Work out the finished part from the listing and answer in its coordinate system (mm). Face numbers are marked on the shaded views. Round coordinates to 2 decimals unless told otherwise and drop trailing zeros. Loops run counter-clockwise (first coordinate to the right, second up) from the corner with the lowest first, then second, coordinate; pieces in that order, holes last. Notation, with made-up numbers: (69.5, -38.5) -> (107.5, -38.5) arc R19 ccw to (107.5, -33.5) -> close; hole circle Ø11 at (9.25, 20.25). An arc over 180 degrees is marked (long way). Use one line per item in the form item = value.
```python
from build123d import *

# Parameters (mm, degrees)
BASE_FLANGE1_DEPTH = 1.524


# Sheet-metal steps are written as plain solids
with BuildPart() as part:
    # Sketch1 → Base-Flange1 (new body)
    with BuildSketch(Plane.XY):
        with BuildLine():
            Line((231.694733782, 24.263932463), (226.322343195, 34.826415896))
            Line((226.322343195, 34.826415896), (224.963957286, 34.135500761))
            Line((224.963957286, 34.135500761), (230.310366707, 23.62409806))
            ThreePointArc((230.310366707, 23.62409806), (229.903279587, 23.531939933), (229.489552508, 23.476777012))
            ThreePointArc((229.489552508, 23.476777012), (228.197526273, 23.373669283), (226.906388141, 23.487358857))
            ThreePointArc((226.906388141, 23.487358857), (226.4596517, 23.740258206), (226.274712745, 24.219141398))
            ThreePointArc((226.274712745, 24.219141398), (224.015809297, 32.216773888), (218.195630565, 38.14891429))
            ThreePointArc((218.195630565, 38.14891429), (220.465583992, 33.0404298), (219.538231847, 27.527778863))
            ThreePointArc((219.538231847, 27.527778863), (216.207783845, 29.677782654), (213.263726879, 32.332387856))
            ThreePointArc((213.263726879, 32.332387856), (210.198099549, 36.324777472), (208.004537358, 40.855288557))
            ThreePointArc((208.004537358, 40.855288557), (206.39770053, 42.404093827), (204.188624103, 42.08675537))
            ThreePointArc((204.188624103, 42.08675537), (201.624892341, 39.331988443), (200.505863828, 35.739045838))
            ThreePointArc((200.505863828, 35.739045838), (199.871363088, 34.249097505), (198.465439283, 33.445408832))
            ThreePointArc((198.465439283, 33.445408832), (196.924665159, 33.149450023), (195.38095855, 32.869188678))
            Line((195.38095855, 32.869188678), (182.741679906, 38.523729549))
            Line((182.741679906, 38.523729549), (182.119318407, 37.132599733))
            Line((182.119318407, 37.132599733), (192.663920738, 32.415171901))
            ThreePointArc((192.663920738, 32.415171901), (161.242789348, 30.704605569), (130.128998565, 35.41051229))
            ThreePointArc((130.128998565, 35.41051229), (113.063651794, 32.366088022), (95.747230087, 33.163658602))
            Line((95.747230087, 33.163658602), (108.559818137, 38.14891429))
            Line((108.559818137, 38.14891429), (108.007201374, 39.569192683))
            Line((108.007201374, 39.569192683), (92.863162197, 33.67679162))
            ThreePointArc((92.863162197, 33.67679162), (86.261009295, 35.281159538), (79.823408008, 37.453648673))
            ThreePointArc((79.823408008, 37.453648673), (78.22024482, 39.499195708), (79.254639852, 41.883398257))
            ThreePointArc((79.254639852, 41.883398257), (82.921318742, 44.978245875), (86.072618329, 48.596522643))
            ThreePointArc((86.072618329, 48.596522643), (95.542941515, 59.597739927), (107.212145233, 68.231596978))
            Line((107.212145233, 68.231596978), (107.212145233, 59.777231813))
            Line((107.212145233, 59.777231813), (108.736145233, 59.777231813))
            Line((108.736145233, 59.777231813), (108.736145233, 69.088203695))
            ThreePointArc((108.736145233, 69.088203695), (116.359031122, 72.623035129), (124.373136037, 75.148415287))
            ThreePointArc((124.373136037, 75.148415287), (131.602965043, 78.776561047), (139.163891612, 81.651671224))
            Line((139.163891612, 81.651671224), (139.163891612, 59.777231813))
            Line((139.163891612, 59.777231813), (140.687891612, 59.777231813))
            Line((140.687891612, 59.777231813), (140.687891612, 82.127226165))
            ThreePointArc((140.687891612, 82.127226165), (157.500365841, 85.268581792), (174.595729834, 84.743286803))
            Line((174.595729834, 84.743286803), (174.595729834, 59.777231813))
            Line((174.595729834, 59.777231813), (176.119729834, 59.777231813))
            Line((176.119729834, 59.777231813), (176.119729834, 84.515885394))
            ThreePointArc((176.119729834, 84.515885394), (185.904383104, 82.318759277), (195.334831423, 78.907975308))
            ThreePointArc((195.334831423, 78.907975308), (199.345089693, 76.463216465), (203.426624103, 74.139406221))
            Line((203.426624103, 74.139406221), (203.426624103, 59.777231813))
            Line((203.426624103, 59.777231813), (204.950624103, 59.777231813))
            Line((204.950624103, 59.777231813), (204.950624103, 73.312546377))
            ThreePointArc((204.950624103, 73.312546377), (209.623865484, 70.909977098), (214.374828712, 68.665011052))
            ThreePointArc((214.374828712, 68.665011052), (206.4297978, 85.930083199), (193.631366333, 99.980221435))
            ThreePointArc((193.631366333, 99.980221435), (209.362770136, 85.826652744), (218.735162472, 66.854071628))
            ThreePointArc((218.735162472, 66.854071628), (224.318551803, 63.708956455), (229.084465035, 59.425026374))
            ThreePointArc((229.084465035, 59.425026374), (222.842822588, 77.340987602), (210.010472895, 91.314912193))
            ThreePointArc((210.010472895, 91.314912193), (225.977718367, 75.717609631), (232.680835608, 54.426837112))
            ThreePointArc((232.680835608, 54.426837112), (233.094865862, 53.67572934), (233.486730489, 52.912823022))
            Line((233.486730489, 52.912823022), (227.814771071, 49.235924899))
            Line((227.814771071, 49.235924899), (228.643767466, 47.957120387))
            Line((228.643767466, 47.957120387), (234.133478106, 51.515874121))
            ThreePointArc((234.133478106, 51.515874121), (236.523898696, 39.310516196), (233.635048327, 27.213433234))
            ThreePointArc((233.635048327, 27.213433234), (232.956717504, 25.546706257), (231.694733782, 24.263932463))
        make_face()
    extrude(amount=-BASE_FLANGE1_DEPTH)


solid = part.part
```
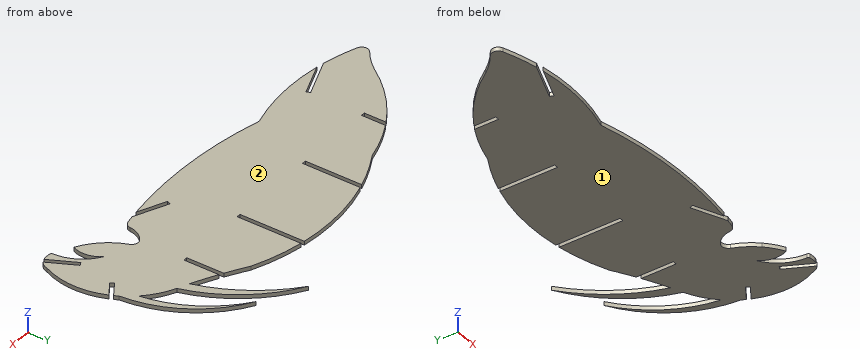
(1) Find section A-A, the plane x = 102. Write down the section's boundary in (y, z).
Completed:
outline = (32.43, -1.52) -> (35.6, -1.52) -> (35.6, 0) -> (32.43, 0) -> close; (37.23, -1.52) -> (64.87, -1.52) -> (64.87, 0) -> (37.23, 0) -> close
(2) Given P1, Ø0.5, axis at y = 76, z = -0.5, coming from the -X side; P2, Ø0.5, axis at x = 139.5, z = -1, coming from the +Y side; P3, Ø0.8, axis at y = 70.5, z = -0.5, coming from the +X side, each flat-ended and moving along its own axis, determine where each tip first touches the part or whether it passes through.
Completed:
P1 = 125.45
P2 = 59.78
P3 = 228.92
(3) Find section B-B, the plane y = 44. Write down the section's boundary in (x, z).
Completed:
outline = (81.88, -1.52) -> (236.24, -1.52) -> (236.24, 0) -> (81.88, 0) -> close
(4) Consider L1, parallel to X at y = 68, z = -0.7; L2, parallel to X at y = 50, z = -0.7; L3, parallel to X at y = 41, z = -1.05. Determine where each line is inside the solid, lowest interval first.
Completed:
L1 = 106.82 to 107.21, 108.74 to 139.16, 140.69 to 174.6, 176.12 to 203.43, 204.95 to 218.41, 227.12 to 229.77
L2 = 87.06 to 228.99, 231.8 to 234.74
L3 = 78.49 to 202.89, 207.95 to 236.51
(5) For a pull along Z with two mould halves and no side action, classify the marked faces 1 and 2 as +Z half, -Z half, draft (parallel to the pull), parting line (faces both ways), or undercut.
Completed:
face_1 = -Z half
face_2 = +Z half
(6) Find section C-C, the plane x = 146. Write down the section's boundary in (y, z).
Completed:
outline = (32.2, -1.52) -> (83.53, -1.52) -> (83.53, 0) -> (32.2, 0) -> close
